Autodesk Fusion 360 part; units mm, degrees
sketch "Sketch1" plane through (0, 0, 0) normal (0, 0, 1) x (1, 0, 0)
  line L0 (3.6667, 54.4476) -> (106.5667, 54.4476)
  line L1 (106.5667, 54.4476) -> (106.5667, -7.3524)
  line L2 (106.5667, -7.3524) -> (3.6667, -7.3524)
  line L3 (3.6667, -7.3524) -> (3.6667, 54.4476)
  line L4 (3.6667, 23.5476) -> (106.5667, 23.5476) construction
  line L5 (3.6667, 28.5476) -> (-0.0333, 28.5476)
  line L6 (-1.3333, 27.2476) -> (-1.3333, 19.8476)
  line L7 (-0.0333, 18.5476) -> (3.6667, 18.5476)
  line L8 (3.6667, 18.5476) -> (3.6667, 28.5476)
  arc A0 (-0.0333, 28.5476) -> (-1.3333, 27.2476) centre (-0.0333, 27.2476) ccw
  arc A1 (-1.3333, 19.8476) -> (-0.0333, 18.5476) centre (-0.0333, 19.8476) ccw
  line L9 (101.5667, 54.4476) -> (106.5667, 54.4476)
  line L10 (106.5667, 54.4476) -> (106.5667, 36.9476)
  line L11 (106.5667, 36.9476) -> (101.5667, 36.9476)
  line L12 (101.5667, 36.9476) -> (101.5667, 54.4476)
  point P0 (-1.3333, 28.5476)
  point P1 (-1.3333, 18.5476)
  dimension "d1" = 102.9
  dimension "d2" = 61.8
  dimension "d7" = 10
  dimension "d8" = 5
  dimension "d9" = 1.3
  dimension "d12" = 5
  dimension "d13" = 17.5
extrude "Extrude1" add sketch "Sketch1" along normal blind 1 contours L0 L1 L2 L3 L8 L11 L12 | L3 L5 L6 L7 L8 A0 A1
The model under review builds one solid part; all positions refer to its coordinate system, in mm. Round coordinates to 2 decimals unless told otherwise and drop trailing zeros. Write each loop counter-clockwise with the first axis right and the second up, starting at its lowest first coordinate (ties: lowest second). Pieces come first, ordered by that corner, then holes. Notation, with made-up numbers: (-10.75, -1) - (-0.75, -1) arc R21 ccw to (-0.75, 25) - close; hole circle Ø9 at (88, 11). An arc over 180 degrees is marked (long way). One line per question, with ' | ' between items.
Item 1: To check wall thickness, follow probe 1 along X at (y, z) = (34.5, 0.1); probe 2 along X at (y, z) = (38, 0.5). State the ranges of each line that lie inside material, in increasing order.
Resolved:
probe 1: x = 3.67 to 106.57 | probe 2: x = 3.67 to 101.57
Item 2: Add section C-C, the plane y = 15.5. Give the boundary of the cut face in (x, z).
Resolved:
outline: (3.67, 0) - (106.57, 0) - (106.57, 1) - (3.67, 1) - close
Item 3: For P1, Ø0.5, axis at x = 2, z = 0.5, coming from the -Y side, flat-tipped, find the tip position at first contact; note if it passes through.
Resolved:
P1: stops at y = 18.55
Item 4: Add section A-A, the plane z = 0.75. Give the boundary of the cut face in (x, y).
Resolved:
outline: (-1.33, 19.85) arc R1.3 ccw to (-0.03, 18.55) - (3.67, 18.55) - (3.67, -7.35) - (106.57, -7.35) - (106.57, 36.95) - (101.57, 36.95) - (101.57, 54.45) - (3.67, 54.45) - (3.67, 28.55) - (-0.03, 28.55) arc R1.3 ccw to (-1.33, 27.25) - close
Item 5: Add section B-B, the plane y = 43. Give the boundary of the cut face in (x, z), then the cut area to 3 significant figures.
Resolved:
outline: (3.67, 0) - (101.57, 0) - (101.57, 1) - (3.67, 1) - close | area: 97.9 mm2
